Read the model definition and answer for the solid it produces. Units are mm, in the model's axes. A direction names the side the tool comes from. Coordinates: 2 decimals unless noted, no trailing zeros. Loops run counter-clockwise (first coordinate to the right, second up) from the corner with the lowest first, then second, coordinate; pieces in that order, holes last.
from build123d import *

# Parameters (mm, degrees)
SKETCH1_W          = 16.002
SKETCH1_H          = 55.5498
EXTRUDE1_DEPTH     = 17.4498
FILLET1_R          = 0.381
CUT_EXTRUDE1_DEPTH = 17.002
SKETCH5_R          = 2.5527
CUT_EXTRUDE2_DEPTH = 18.4498


with BuildPart() as part:
    # Sketch1 → Extrude1 (new body)
    with BuildSketch(Plane(origin=(0, 0, 0), x_dir=(1, 0, 0), z_dir=(0, 1, 0))):
        with Locations((8.001, -27.7749)):
            Rectangle(SKETCH1_W, SKETCH1_H)
    extrude(amount=EXTRUDE1_DEPTH)

    # Sketch3 → Cut-Revolve1 (revolve, cut)
    with BuildSketch(Plane(origin=(8.0518, 0, 0), x_dir=(0, 0, -1), z_dir=(1, 0, 0))):
        Polygon((-17.8435, 17.4498), (-17.8435, 9.525), (-15.4686, 9.525), (-15.4686, 6.6548), (-16.941174995, 6.6548), (-17.3482, 0), (-11.0998, 0), (-11.0998, 17.4498), align=None)
    revolve(axis=Axis((8.0518, 31.679444444, 11.0998), (0, -1, 0)), mode=Mode.SUBTRACT)

    # Fillet1
    fillet1_edges = [part.edges().sort_by_distance(p)[0] for p in [
        (8.0518, 6.6548, 5.258425005),
    ]]
    fillet(fillet1_edges, radius=FILLET1_R)

    # Sketch4 → Cut-Extrude1 (cut, through all)
    with BuildSketch(Plane(origin=(16.002, 0, 0), x_dir=(0, 0, -1), z_dir=(1, 0, 0))):
        Polygon((-55.5498, 6.97992), (-55.5498, 17.4498), (-24.5872, 17.4498), align=None)
    extrude(amount=-CUT_EXTRUDE1_DEPTH, mode=Mode.SUBTRACT)

    # Sketch5 → Cut-Extrude2 (cut, through all)
    with BuildSketch(Plane.XZ):
        with Locations(Location((8.0518, 49.1998, 0), (0, 0, 270))):  # turned: the seam where the file's is
            Circle(SKETCH5_R)
    extrude(amount=-CUT_EXTRUDE2_DEPTH, mode=Mode.SUBTRACT)


solid = part.part
Q1. Flat-ended cylindrical pins translate along their axes: pin 1 Ø4 at (x, z) = (11.5, 11) entering from +Y (3 decimals); pin 2 Ø6 at (x, z) = (5.5, 49) entering from +Y. Find the tip coordinate at first contact, or state that the pin passes through.
Findings below:
pin 1: stops at y = 9.525
pin 2: stops at y = 10.21
Q2. A cutting plane is placed at D-D (z = 27). Give the vertices of the cut face in (x, y), then the cut area to 3 significant figures.
Findings below:
outline: (0, 0) - (16, 0) - (16, 16.63) - (0, 16.63) - close
area: 266 mm2
Q3. Determine the mould class of faces 4 (the face through (16.002, 7, 22)), 5 (the face through (8, 9, 0)), 6 (the face through (7.755, 13.432, 4.363)), 7 (the face through (0, 7, 22)) for opening direction X: +X half, -X half, draft (parallel to the pull), parting line (faces both ways), or undercut.
Findings below:
face 4: +X half
face 5: draft
face 6: undercut
face 7: -X half
Q4. A cutting plane is placed at A-A (y = 5). Give the vertices of the cut face in (x, z).
Findings below:
outline: (0, 0) - (16, 0) - (16, 55.55) - (0, 55.55) - close; hole circle Ø11.89 at (8.05, 11.1); hole circle Ø5.11 at (8.05, 49.2)
Q5. A cutting plane is placed at B-B (x = 6.5). Count the separate pieces of the cut face and the enclosed holes in it, then the cut area to 3 significant figures.
Findings below:
separate pieces: 3
enclosed holes: 0
area: 565 mm2
Q6. A cutting plane is placed at C-C (y = 14.25). Give the vertices of the cut face in (x, z), then the cut area to 3 significant figures.
Findings below:
outline: (0, 0) - (16, 0) - (16, 34.05) - (0, 34.05) - close; hole circle Ø13.49 at (8.05, 11.1)
area: 402 mm2
Q7. Which of the six approach directions +Z, -Z, +X, -X, +Y, -Y give full straight-line access (tool end or side, diameter ignored) to faces 1 (the face through (8, 9.525, 16)), 2 (the face through (12.1, 6.655, 13.2)), 3 (the face through (6, 17.45, 18))?
Findings below:
face 1: +Y
face 2: -Y
face 3: +Z, -Z, +X, -X, +Y
Q8. Straight lines are drawn through the part: probe 1 along Z at (x, y) = (8.75, 3); probe 2 along Z at (x, y) = (7, 3); probe 3 along Y at (x, z) = (6.5, 16) (3 decimals). For each, find the intervals that lie inside material, in ascending order.
Findings below:
probe 1: z = 0 to 5.08, 17.12 to 46.74, 51.66 to 55.55
probe 2: z = 0 to 5.13, 17.07 to 46.87, 51.53 to 55.55
probe 3: y = 6.655 to 9.525
